Can you work these out from the model? Positions are in its coordinate system, mm. Face numbers are marked on the shaded views. A direction names the side the tool comes from. Coordinates: 2 decimals unless noted, no trailing zeros. Order: outer loops, then holes, each group sorted by start corner. A loop starts at its lowest first (then second) coordinate and runs counter-clockwise, first axis right, second up. Notation, with made-up numbers: (31.5, -29) -> (75.5, -29) arc R16 cw to (75.5, -1) -> close; hole circle Ø4 at (44.5, 65.5). An arc over 180 degrees is marked (long way). Answer as CSV lines item,"result".
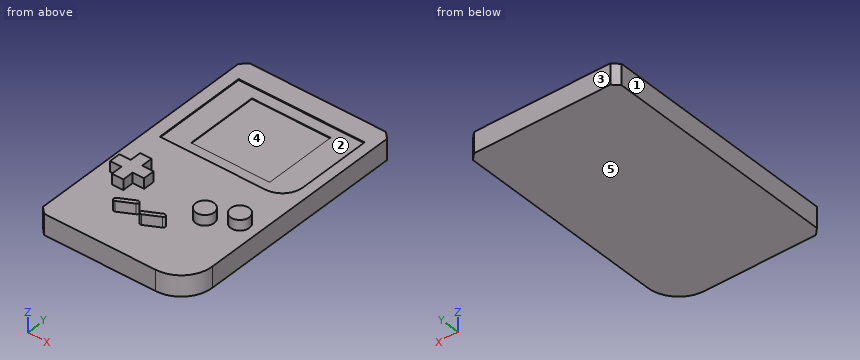
from build123d import *

# Parameters (mm, degrees)
SKETCH_1_R       = 4.5
EXTRUDE_10_DEPTH = 10
SKETCH_1_15_W    = 38
SKETCH_1_15_H    = 35.5
EXTRUDE_11_DEPTH = 9.5
SKETCH_1_16_W    = 38
SKETCH_1_16_H    = 35.5
EXTRUDE_12_DEPTH = 9.2
SKETCH_1_17_R    = 4.5
EXTRUDE_13_DEPTH = 15


with BuildPart() as part:
    # Sketch 1 → Extrude 10 (new body)
    with BuildSketch(Plane.XY):
        with BuildLine():
            Line((0, 117), (0, 3))
            Line((0, 3), (3, 0))
            Line((3, 0), (57, 0))
            ThreePointArc((57, 0), (67.606601718, 4.393398282), (72, 15))
            Line((72, 15), (72, 22.5))
            Line((72, 22.5), (72, 42))
            Line((72, 42), (72, 117))
            Line((72, 117), (69, 120))
            Line((69, 120), (3, 120))
            Line((3, 120), (0, 117))
        make_face()
        with BuildLine():
            ThreePointArc((22.625564011, 17.861279905), (21.273144855, 18.274755935), (21.686620885, 19.627175091))
            Line((21.686620885, 19.627175091), (28.750201628, 23.382947593))
            ThreePointArc((28.750201628, 23.382947593), (30.102620784, 22.969471563), (29.689144754, 21.617052407))
            Line((29.689144754, 21.617052407), (22.625564011, 17.861279905))
        make_face(mode=Mode.SUBTRACT)
        Polygon((10.9884201, 41.001199035), (10.9884201, 46.501199035), (16.4884201, 46.501199035), (16.4884201, 41.001199035), (21.9884201, 41.001199035), (21.9884201, 35.501199035), (16.4884201, 35.501199035), (16.4884201, 30.001199035), (10.9884201, 30.001199035), (10.9884201, 35.501199035), (5.4884201, 35.501199035), (5.4884201, 41.001199035), align=None, mode=Mode.SUBTRACT)
        with BuildLine():
            ThreePointArc((41.530528437, 23.382947593), (42.882947593, 22.969471563), (42.469471563, 21.617052407))
            Line((42.469471563, 21.617052407), (35.40589082, 17.861279905))
            ThreePointArc((35.40589082, 17.861279905), (34.053471664, 18.274755935), (34.466947694, 19.627175091))
            Line((34.466947694, 19.627175091), (41.530528437, 23.382947593))
        make_face(mode=Mode.SUBTRACT)
        with Locations((51, 36)):
            Circle(SKETCH_1_R, mode=Mode.SUBTRACT)
        with Locations((63, 42)):
            Circle(SKETCH_1_R, mode=Mode.SUBTRACT)
        with BuildLine():
            Line((6, 70.706412031), (6, 110))
            Line((6, 110), (67, 110))
            Line((67, 110), (67, 74))
            ThreePointArc((67, 74), (64.071067812, 66.928932188), (57, 64))
            Line((57, 64), (17, 64))
            Line((17, 64), (6, 64))
            Line((6, 64), (6, 70.706412031))
        make_face(mode=Mode.SUBTRACT)
    extrude(amount=EXTRUDE_10_DEPTH)

    # Sketch 1_15 → Extrude 11 (add)
    with BuildSketch(Plane.XY):
        with BuildLine():
            Line((6, 64), (57, 64))
            ThreePointArc((57, 64), (64.071067812, 66.928932188), (67, 74))
            Line((67, 74), (67, 110))
            Line((67, 110), (6, 110))
            Line((6, 110), (6, 64))
        make_face()
        with Locations((36, 86.75)):
            Rectangle(SKETCH_1_15_W, SKETCH_1_15_H, mode=Mode.SUBTRACT)
    extrude(amount=EXTRUDE_11_DEPTH)

    # Sketch 1_16 → Extrude 12 (add)
    with BuildSketch(Plane.XY):
        with Locations((36, 86.75)):
            Rectangle(SKETCH_1_16_W, SKETCH_1_16_H)
    extrude(amount=EXTRUDE_12_DEPTH)

    # Sketch 1_17 → Extrude 13 (add)
    with BuildSketch(Plane.XY):
        Polygon((10.9884201, 46.501199035), (16.4884201, 46.501199035), (16.4884201, 41.001199035), (21.9884201, 41.001199035), (21.9884201, 35.501199035), (16.4884201, 35.501199035), (16.4884201, 30.001199035), (10.9884201, 30.001199035), (10.9884201, 35.501199035), (5.4884201, 35.501199035), (5.4884201, 41.001199035), (10.9884201, 41.001199035), align=None)
        with Locations((51, 36)):
            Circle(SKETCH_1_17_R)
        with Locations((63, 42)):
            Circle(SKETCH_1_17_R)
        with BuildLine():
            Line((22.625564011, 17.861279905), (29.689144754, 21.617052407))
            ThreePointArc((29.689144754, 21.617052407), (30.102620784, 22.969471563), (28.750201628, 23.382947593))
            Line((28.750201628, 23.382947593), (21.686620885, 19.627175091))
            ThreePointArc((21.686620885, 19.627175091), (21.273144855, 18.274755935), (22.625564011, 17.861279905))
        make_face()
        with BuildLine():
            Line((41.530528437, 23.382947593), (34.466947694, 19.627175091))
            ThreePointArc((34.466947694, 19.627175091), (34.053471664, 18.274755935), (35.40589082, 17.861279905))
            Line((35.40589082, 17.861279905), (42.469471563, 21.617052407))
            ThreePointArc((42.469471563, 21.617052407), (42.882947593, 22.969471563), (41.530528437, 23.382947593))
        make_face()
    extrude(amount=EXTRUDE_13_DEPTH)


solid = part.part
Q1. Imagine slicing it at C-C (x = 8). List the corners of the cut face in (y, z) for me.
Solution:
outline,"(0, 0) -> (120, 0) -> (120, 10) -> (110, 10) -> (110, 9.5) -> (64, 9.5) -> (64, 10) -> (41, 10) -> (41, 15) -> (35.5, 15) -> (35.5, 10) -> (0, 10) -> close"
Q2. For P1, Ø1, axis at x = 39.5, z = 4, coming from the -Y side; P2, Ø1.5, axis at y = 32, z = 13, coming from the +X side; P3, Ø2.5, axis at x = 14, z = 11.5, coming from the -Y side; P4, Ø2.5, axis at x = 13, z = 12, coming from the +Y side, each with a flat end and sliding along its axis, tell me the tip position at first contact or that it passes through.
Solution:
P1,"y = 0"
P2,"x = 54.11"
P3,"y = 30"
P4,"y = 46.5"
Q3. We'd pull the mould along Y, two halves only. Please class the marked faces 1, 2 and 3: pulls with the +Y half, pulls with the -Y half, needs draft (parallel to the pull), parting line crosses it, or undercut.
Solution:
face 1,"needs draft"
face 2,"undercut"
face 3,"pulls with the +Y half"
Q4. If I drill on line 1 (Y direction, x = 47, z = 9.25); line 2 (Z direction, x = 17, y = 41.5); line 3 (Z direction, x = 31, y = 74), over which ranges is the centre line in solid material (lowest first)?
Solution:
line 1,"0 to 69, 104.5 to 120"
line 2,"0 to 10"
line 3,"0 to 9.2"
Q5. Imagine slicing it at D-D (x = 38). List the corners of the cut face in (y, z) for me, and give its area (3 significant figures).
Solution:
outline,"(0, 0) -> (120, 0) -> (120, 10) -> (110, 10) -> (110, 9.5) -> (104.5, 9.5) -> (104.5, 9.2) -> (69, 9.2) -> (69, 9.5) -> (64, 9.5) -> (64, 10) -> (21.51, 10) -> (21.51, 15) -> (19.24, 15) -> (19.24, 10) -> (0, 10) -> close"
area,"1,180 mm2"
Q6. Which directions (+Z, -Z, +X, -X, +Y, -Y) give clear straight access to the entire face, cutting with the end or side of a thin tool? Please do the marked faces 4 and 5.
Solution:
face 4,"+Z"
face 5,"-Z, +X, -X, +Y, -Y"
Q7. Imagine slicing it at A-A (z = 12). List the corners of the cut face in (x, y) for me.
Solution:
outline,"(5.49, 35.5) -> (10.99, 35.5) -> (10.99, 30) -> (16.49, 30) -> (16.49, 35.5) -> (21.99, 35.5) -> (21.99, 41) -> (16.49, 41) -> (16.49, 46.5) -> (10.99, 46.5) -> (10.99, 41) -> (5.49, 41) -> close; (21.69, 19.63) arc R1 ccw to (22.63, 17.86) -> (29.69, 21.62) arc R1 ccw to (28.75, 23.38) -> close; (34.47, 19.63) arc R1 ccw to (35.41, 17.86) -> (42.47, 21.62) arc R1 ccw to (41.53, 23.38) -> close; circle Ø9 at (51, 36); circle Ø9 at (63, 42)"
Q8. Imagine slicing it at B-B (y = 101). List the corners of the cut face in (x, z) for me, and give its area (3 significant figures).
Solution:
outline,"(0, 0) -> (72, 0) -> (72, 10) -> (67, 10) -> (67, 9.5) -> (55, 9.5) -> (55, 9.2) -> (17, 9.2) -> (17, 9.5) -> (6, 9.5) -> (6, 10) -> (0, 10) -> close"
area,"678 mm2"
